```python
from build123d import *

# Parameters (mm, degrees)
RESSALTO_EXTRUS_O1_DEPTH      = 280
RESSALTO_EXTRUS_O1_DEPTH_BACK = 10
ESBO_O1_R                     = 10
ESBO_O2_R                     = 7.5
CORTE_EXTRUS_O1_DEPTH         = 280
RESSALTO_EXTRUS_O2_DEPTH      = 10
RESSALTO_EXTRUS_O2_DEPTH_BACK = 10
ESBO_O4_W                     = 20
ESBO_O4_H                     = 20
CORTE_EXTRUS_O2_DEPTH         = 10
CORTE_EXTRUS_O2_DEPTH_BACK    = 10
ESBO_O3_R                     = 2.5


with BuildPart() as part:
    # Esboço1 → Ressalto-extrusão1 (new, two sides: drawn at the far end of the back side and taken through both)
    with BuildSketch(Plane.XY.offset(-RESSALTO_EXTRUS_O1_DEPTH_BACK)):
        Circle(ESBO_O1_R)
    extrude(amount=RESSALTO_EXTRUS_O1_DEPTH + RESSALTO_EXTRUS_O1_DEPTH_BACK)

    # Esboço2 → Corte-extrusão1 (cut)
    with BuildSketch(Plane.XY):
        Circle(ESBO_O2_R)
    extrude(amount=CORTE_EXTRUS_O1_DEPTH, mode=Mode.SUBTRACT)

    # Esboço4 → Ressalto-extrusão2 (add, two sides: drawn at the far end of the back side and taken through both)
    with BuildSketch(Plane.XY.offset(-RESSALTO_EXTRUS_O2_DEPTH_BACK)):
        Rectangle(ESBO_O4_W, ESBO_O4_H)
    extrude(amount=RESSALTO_EXTRUS_O2_DEPTH + RESSALTO_EXTRUS_O2_DEPTH_BACK)

    # Esboço3 → Corte-extrusão2 (cut, two sides: drawn at the far end of the back side and taken through both)
    with BuildSketch(Plane(origin=(0, 0, 0), x_dir=(0, 0, -1), z_dir=(1, 0, 0)).offset(-CORTE_EXTRUS_O2_DEPTH_BACK)):
        Circle(ESBO_O3_R)
    extrude(amount=CORTE_EXTRUS_O2_DEPTH + CORTE_EXTRUS_O2_DEPTH_BACK, mode=Mode.SUBTRACT)


solid = part.part
```
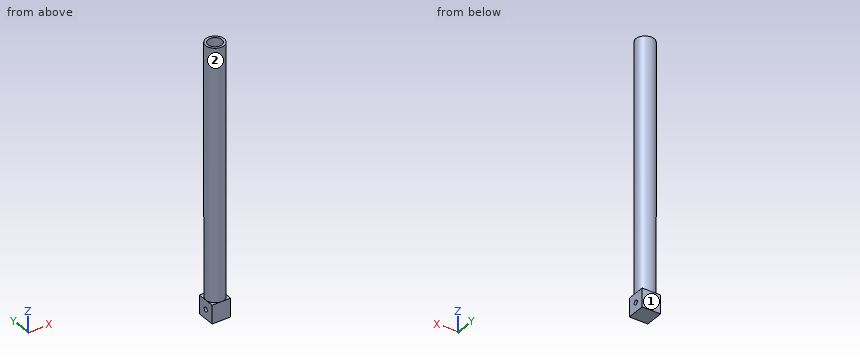
Geometry: final body of the model. Coordinates: model frame, mm. Face numbers are marked on the shaded views. A direction names the side the tool comes from. Coordinates: 2 decimals unless noted, no trailing zeros. Order: outer loops, then holes, each group sorted by start corner. A loop starts at its lowest first (then second) coordinate and runs counter-clockwise, first axis right, second up. Notation, with made-up numbers: M 63,-38.75 L 76,-38.75 A20 ccw 76,-20.75 Z; hole C 58,-4 d11. An arc over 180 degrees is marked long. Answer as CSV lines item,"result".
Q1. Section C-C on z = 88.5. Return the cut outline in (x, y), and give its area (3 significant figures).
Answers:
outline,"C 0,0 d20; hole C 0,0 d15"
area,"137 mm^2"
Q2. Line query: probe 1 along X at (y, z) = (0, 135.5); probe 2 along Y at (x, z) = (5, 0); probe 3 along Z at (x, y) = (0.25, -6.5). Output: solid intervals per line, ascending. Write a range as [from, to].
Answers:
probe 1,"x = [-10, -7.5], [7.5, 10]"
probe 2,"y = [-10, -2.5], [2.5, 10]"
probe 3,"z = [-10, 10]"
Q3. First-contact query: P1, Ø1, axis at x = -5.5, z = 196.5, coming from the -Y side; P2, Ø6, axis at x = -3.5, z = 239.5, coming from the +Y side; P3, Ø3, axis at x = -4.5, z = 183, coming from the -Y side. Flat tips, straight axial feed; report the tip coordinate or a pass-through.
Answers:
P1,"stops at y = -8.66"
P2,"stops at y = 9.99"
P3,"stops at y = -9.54"
Q4. Section B-B on x = 4.75. Return the cut outline in (y, z).
Answers:
outline,"M -10,-10 L 10,-10 L 10,10 L 8.8,10 L 8.8,280 L 5.8,280 L 5.8,10 L -5.8,10 L -5.8,280 L -8.8,280 L -8.8,10 L -10,10 Z; hole C 0,0 d5"
Q5. Section A-A on z = 0. Return the cut outline in (x, y), and give its area (3 significant figures).
Answers:
outline,"M -10,-10 L 10,-10 L 10,-2.5 L -10,-2.5 Z; M -10,2.5 L 10,2.5 L 10,10 L -10,10 Z"
area,"300 mm^2"
Q6. Set-up query: the marked faces 1 and 2. Return all of +Z, -Z, +X, -X, +Y, -Y with unobstructed straight access to the full face (end or side cutting, diameter ignored); none if empty.
Answers:
face 1,"+Z, -Z, +X, -X, +Y"
face 2,"+Z"
